from build123d import *

# Parameters (mm, degrees)
SKETCH1_R           = 4
BOSS_EXTRUDE1_DEPTH = 5


with BuildPart() as part:
    # Sketch1 → Boss-Extrude1 (new body)
    with BuildSketch(Plane.XY):
        Polygon((-10, 80), (-10, -20), (-10, -25), (-5, -25), (-5, -20), (-1.5, -20), (-1.5, -17), (-2.6, -17), (-2.6, -14.7), (-1.5, -14.7), (-1.5, -10), (1.5, -10), (1.5, -14.7), (2.6, -14.7), (2.6, -17), (1.5, -17), (1.5, -20), (5, -20), (5, -25), (10, -25), (10, -20), (10, 80), (10, 85), (5, 85), (5, 80), (1.5, 80), (1.5, 77), (2.6, 77), (2.6, 74.7), (1.5, 74.7), (1.5, 70), (-1.5, 70), (-1.5, 74.7), (-2.6, 74.7), (-2.6, 77), (-1.5, 77), (-1.5, 80), (-5, 80), (-5, 85), (-10, 85), align=None)
        with Locations((0, 5)):
            Circle(SKETCH1_R, mode=Mode.SUBTRACT)
    extrude(amount=BOSS_EXTRUDE1_DEPTH)


solid = part.part
CAD build for the part. Positions are in the model's coordinates, mm. A direction names the side the tool comes from. Round coordinates to 2 decimals unless told otherwise and drop trailing zeros. Loops run counter-clockwise (first coordinate to the right, second up) from the corner with the lowest first, then second, coordinate; pieces in that order, holes last. Notation, with made-up numbers: M 61,73 L 90,73 A31 cw 90,109 Z; hole C 65.25,81.25 d4. An arc over 180 degrees is marked long. One line per question, with ' | ' between items. Start each with the question number.
Item 1: Cut at A-A, the plane x = 0. Write the cut outline in (y, z), plus the area to 3 significant figures.
Item 2: Which spindle directions (+Z, -Z, +X, -X, +Y, -Y) get a long thin tool onto all of the face, cutting with end or side? Do faces 4 (the flat face through (1.5, -18, 2)), 5 (the flat face through (2.6, 76, 2)), 6 (the flat face through (-1.5, 78, 2)). Say none if no direction does.
Item 3: Wall check: line 1 (X direction, y = 72.5, z = 0.5); line 2 (Y direction, x = 0, z = 3.75); line 3 (Y direction, x = 4.5, z = 1.2). Give the ranges that are in metal, low to high.
Item 4: Pin check, flat tips, straight feed: pin 1 Ø1.2 at (x, z) = (2, 2) entering from +Y; pin 2 Ø0.9 at (x, z) = (2, 2.5) entering from -Y. Stop position of each tip, or through.
Item 5: Two-plate mould, pull along X, no slides. Class faces 1 (the flat face through (-10, 31, 2)), 2 (the flat face through (0, 31, 0)), 3 (the flat face through (5, 83, 2)): pulls with the +X half, pulls with the -X half, needs draft (parallel to the pull), parting line crosses it, or undercut.
Item 6: Cut at B-B, the plane y = 5. Write the cut outline in (x, z).
Responses:
1) outline: M -10,0 L 1,0 L 1,5 L -10,5 Z; M 9,0 L 70,0 L 70,5 L 9,5 Z | area: 360 mm²
2) face 4: +Z, -Z, -Y | face 5: +Z, -Z | face 6: +Z, -Z, +Y
3) line 1: x = -10 to -1.5, 1.5 to 10 | line 2: y = -10 to 1, 9 to 70 | line 3: y = -20 to 80
4) pin 1: stops at y = 80 | pin 2: stops at y = -20
5) face 1: pulls with the -X half | face 2: needs draft | face 3: undercut
6) outline: M -10,0 L -4,0 L -4,5 L -10,5 Z; M 4,0 L 10,0 L 10,5 L 4,5 Z
